Can you work these out from the model? Positions are in its coordinate system, mm. Face numbers are marked on the shaded views. A direction names the side the tool comes from. Give positions to 0.01 mm unless a question says otherwise; leave off trailing zeros. Order: outer loops, then holes, each group sorted by start corner. A loop starts at its lowest first (then second) coordinate and runs counter-clockwise, first axis right, second up. Notation, with made-up numbers: M 7,-9.5 L 39,-9.5 A20 ccw 39,18.5 Z; hole C -23.5,38 d7. An arc over 180 degrees is marked long. One line per question, with ' | ' between items. Start each with the question number.
1) For the marked faces 1, 2 and 3, which set-ups out of +Z, -Z, +X, -X, +Y, -Y let a thin tool reach every point of the face, with its end or its side?
2) If we section it at C-C, the plane z = -27.5: Please give me the cut outline in (x, y).
3) Thinking about a two-plate mould opening in Y: for the marked faces 4, 5, 6 and 7, which applies, +Y half, -Y half, draft (parallel to the pull), parting line (faces both ways), or undercut?
4) Please list where these lines run through material, in increasing order: line 1 along Z through (x, y) = (18.5, 0); line 2 along X through (y, z) = (-0.5, -13); line 3 along Y through (x, z) = (0, -35). Write a range as [from, to].
5) If we section it at A-A, the plane y = 0: Please give me the cut outline in (x, z).
6) I'm going to push flat-ended pins straight in: pin 1 Ø5 at (y, z) = (-7.5, -23) entering from -X; pin 2 Ø5 at (y, z) = (13.5, -29) entering from +X; pin 3 Ø7 at (x, y) = (3.5, 5) entering from +Z; pin 4 Ø6 at (x, y) = (-11, 6) entering from +Z. Where does each tip first touch, or does it pass through?
7) If we section it at B-B, the plane z = -19: Please give me the cut outline in (x, y).
8) If we section it at D-D, the plane x = 0: Please give me the cut outline in (y, z), plus the area to 3 significant figures.
```python
from build123d import *

# Parameters (mm, degrees)
SKETCH3_R               = 19.05
BOSS_EXTRUDE1_DEPTH     = 38.1
CUT_EXTRUDE2_DEPTH      = 25.4
CUT_EXTRUDE4_DEPTH      = 20.32
SKETCH11_R              = 12.732490025
CUT_EXTRUDE5_DEPTH      = 3.81
SKETCH12_R              = 11.742927305
CUT_EXTRUDE6_DEPTH      = 1.016
FILLET2_R               = 0.508
CUT_EXTRUDE7_DEPTH      = 47.6627796
CUT_EXTRUDE7_DEPTH_BACK = 47.6627796
SKETCH14_R              = 5.08


with BuildPart() as part:
    # Sketch3 → Boss-Extrude1 (new body)
    with BuildSketch(Plane.XY):
        Circle(SKETCH3_R)
    extrude(amount=-BOSS_EXTRUDE1_DEPTH)

    # Sketch6 → Cut-Extrude2 (cut)
    with BuildSketch(Plane(origin=(0, 0, -38.1), x_dir=(-1, 0, 0), z_dir=(0, 0, -1))):
        with BuildLine():
            Line((4.445692932, 13.555581222), (-4.445692932, 13.555581222))
            Line((-4.445692932, 13.555581222), (-4.445692932, 16.13135994))
            Line((-4.445692932, 16.13135994), (-7.735378966, 16.13135994))
            ThreePointArc((-7.735378966, 16.13135994), (-17.89013307, 0), (-7.735378966, -16.13135994))
            Line((-7.735378966, -16.13135994), (-4.445692932, -16.13135994))
            Line((-4.445692932, -16.13135994), (-4.445692932, -13.555581222))
            Line((-4.445692932, -13.555581222), (4.445692932, -13.555581222))
            Line((4.445692932, -13.555581222), (4.445692932, -16.13135994))
            Line((4.445692932, -16.13135994), (7.735378966, -16.13135994))
            ThreePointArc((7.735378966, -16.13135994), (17.89013307, 0), (7.735378966, 16.13135994))
            Line((7.735378966, 16.13135994), (4.445692932, 16.13135994))
            Line((4.445692932, 16.13135994), (4.445692932, 13.555581222))
        make_face()
    extrude(amount=-CUT_EXTRUDE2_DEPTH, mode=Mode.SUBTRACT)

    # Sketch10 → Cut-Extrude4 (cut)
    with BuildSketch(Plane(origin=(0, 0, -38.1), x_dir=(-1, 0, 0), z_dir=(0, 0, -1))):
        with BuildLine():
            Line((-8.382, 17.106857572), (8.382, 17.106857572))
            ThreePointArc((8.382, 17.106857572), (0, 19.054089968), (-8.382, 17.106857572))
        make_face()
        with BuildLine():
            Line((-8.382, -17.106857572), (8.382, -17.106857572))
            ThreePointArc((8.382, -17.106857572), (0, -19.054089968), (-8.382, -17.106857572))
        make_face()
    extrude(amount=-CUT_EXTRUDE4_DEPTH, mode=Mode.SUBTRACT)

    # Sketch11 → Cut-Extrude5 (cut)
    with BuildSketch(Plane.XY):
        Circle(SKETCH11_R)
    extrude(amount=-CUT_EXTRUDE5_DEPTH, mode=Mode.SUBTRACT)

    # Sketch12 → Cut-Extrude6 (cut)
    with BuildSketch(Plane.XY.offset(-3.81)):
        Circle(SKETCH12_R)
    extrude(amount=-CUT_EXTRUDE6_DEPTH, mode=Mode.SUBTRACT)

    # Fillet2
    fillet2_edges = [part.edges().sort_by_distance(p)[0] for p in [
        (-11.742927305, 0, -3.81),
    ]]
    fillet(fillet2_edges, radius=FILLET2_R)

    # Sketch14 → Cut-Extrude7 (cut, two sides: drawn at the far end of the back side and taken through both)
    with BuildSketch(Plane(origin=(0, 0, 0), x_dir=(0, 0, -1), z_dir=(1, 0, 0)).offset(-CUT_EXTRUDE7_DEPTH_BACK)):
        with Locations((27.94, 0)):
            Circle(SKETCH14_R)
    extrude(amount=CUT_EXTRUDE7_DEPTH + CUT_EXTRUDE7_DEPTH_BACK, mode=Mode.SUBTRACT)


solid = part.part
```
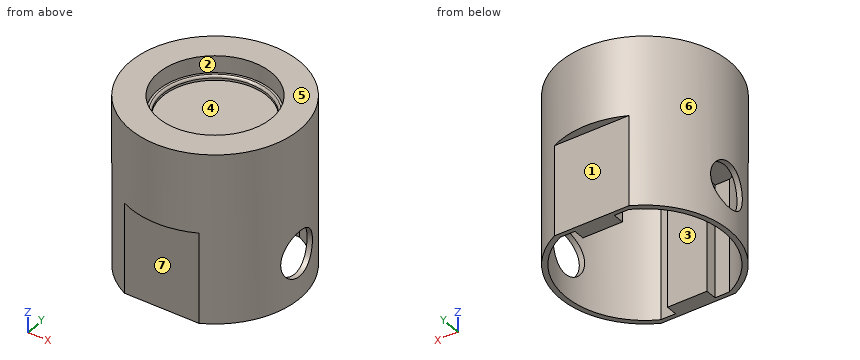
Results found:
1) face 1: -Z, +X, -X, +Y | face 2: +Z | face 3: -Z
2) outline: M -18.37,-5.06 A19.05 ccw -8.38,-17.11 L 8.38,-17.11 A19.05 ccw 18.37,-5.06 L 17.16,-5.06 A17.89 cw 7.74,-16.13 L 4.45,-16.13 L 4.45,-13.56 L -4.45,-13.56 L -4.45,-16.13 L -7.74,-16.13 A17.89 cw -17.16,-5.06 Z; M -18.37,5.06 L -17.16,5.06 A17.89 cw -7.74,16.13 L -4.45,16.13 L -4.45,13.56 L 4.45,13.56 L 4.45,16.13 L 7.74,16.13 A17.89 cw 17.16,5.06 L 18.37,5.06 A19.05 ccw 8.38,17.11 L -8.38,17.11 A19.05 ccw Z
3) face 4: undercut | face 5: draft | face 6: parting line | face 7: -Y half
4) line 1: z = [-38.1, -33.02], [-22.86, 0] | line 2: x = [-19.04, -17.88], [17.88, 19.04] | line 3: y = [-17.11, -13.56], [13.56, 17.11]
5) outline: M -19.05,-38.1 L -17.89,-38.1 L -17.89,-33.02 L -19.05,-33.02 Z; M -19.05,-22.86 L -17.89,-22.86 L -17.89,-12.7 L 17.89,-12.7 L 17.89,-22.86 L 19.05,-22.86 L 19.05,0 L 12.73,0 L 12.73,-3.81 L 12.25,-3.81 A0.51 ccw 11.74,-4.32 L 11.74,-4.83 L -11.74,-4.83 L -11.74,-4.32 A0.51 ccw -12.25,-3.81 L -12.73,-3.81 L -12.73,0 L -19.05,0 Z; M 17.89,-38.1 L 19.05,-38.1 L 19.05,-33.02 L 17.89,-33.02 Z
6) pin 1: stops at x = -18.38 | pin 2: stops at x = 15.55 | pin 3: stops at z = -4.83 | pin 4: stops at z = 0
7) outline: M -8.38,-17.11 L 8.38,-17.11 A19.05 ccw 8.38,17.11 L -8.38,17.11 A19.05 ccw Z; hole M -7.74,-16.13 L -4.45,-16.13 L -4.45,-13.56 L 4.45,-13.56 L 4.45,-16.13 L 7.74,-16.13 A17.89 ccw 7.74,16.13 L 4.45,16.13 L 4.45,13.56 L -4.45,13.56 L -4.45,16.13 L -7.74,16.13 A17.89 ccw Z
8) outline: M -19.05,-17.78 L -17.11,-17.78 L -17.11,-38.1 L -13.56,-38.1 L -13.56,-12.7 L 13.56,-12.7 L 13.56,-38.1 L 17.11,-38.1 L 17.11,-17.78 L 19.05,-17.78 L 19.05,0 L 12.73,0 L 12.73,-3.81 L 12.25,-3.81 A0.51 ccw 11.74,-4.32 L 11.74,-4.83 L -11.74,-4.83 L -11.74,-4.32 A0.51 ccw -12.25,-3.81 L -12.73,-3.81 L -12.73,0 L -19.05,0 Z | area: 563 mm²
